Geometry check sheet. Reference: drawing and pictorial views, mm from the part's lowest x, y, z. A direction names the side the tool comes from. Coordinates: 2 decimals unless noted, no trailing zeros. Loops run counter-clockwise (first coordinate to the right, second up) from the corner with the lowest first, then second, coordinate; pieces in that order, holes last. Notation, with made-up numbers: (50.5, 57) -> (105.5, 57) arc R14 cw to (105.5, 84) -> close; hole circle Ø2 at (0, 59). An arc over 180 degrees is marked (long way). Answer as a JSON object with one key per item and string values.
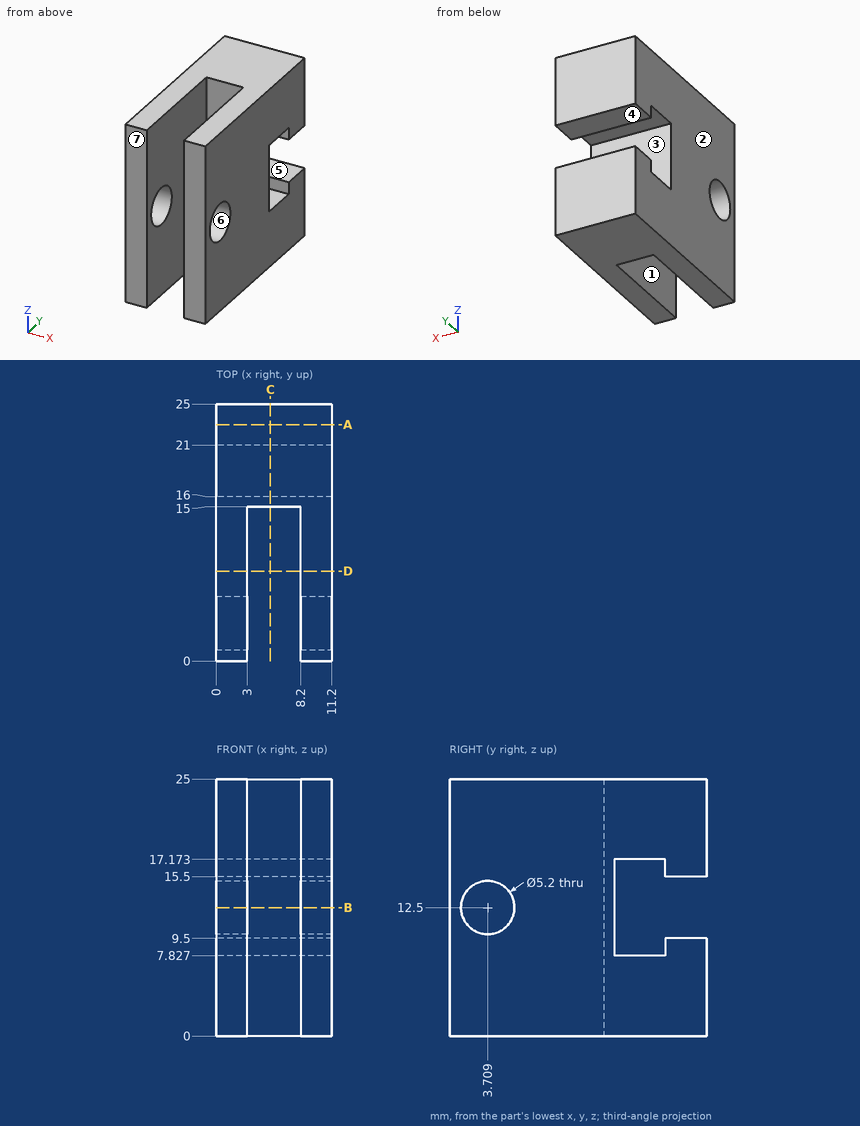
1. Section check B-B, the plane z = 12.5. Record the boundary of the cut face in (x, y), then the cut area to 3 significant figures.
Evaluation:
{"outline": "(0, 0) -> (3, 0) -> (3, 1.11) -> (0, 1.11) -> close; (0, 6.31) -> (3, 6.31) -> (3, 15) -> (8.2, 15) -> (8.2, 6.31) -> (11.2, 6.31) -> (11.2, 16) -> (0, 16) -> close; (8.2, 0) -> (11.2, 0) -> (11.2, 1.11) -> (8.2, 1.11) -> close", "area": "70.0 mm^2"}
2. Section check D-D, the plane y = 8.75. Record the boundary of the cut face in (x, z), then the cut area to 3 significant figures.
Evaluation:
{"outline": "(0, 0) -> (3, 0) -> (3, 25) -> (0, 25) -> close; (8.2, 0) -> (11.2, 0) -> (11.2, 25) -> (8.2, 25) -> close", "area": "150 mm^2"}
3. Section check A-A, the plane y = 23. Record the boundary of the cut face in (x, z).
Evaluation:
{"outline": "(0, 0) -> (11.2, 0) -> (11.2, 9.5) -> (0, 9.5) -> close; (0, 15.5) -> (11.2, 15.5) -> (11.2, 25) -> (0, 25) -> close"}
4. Section check C-C, the plane x = 5.25. Record the boundary of the cut face in (y, z), then the cut area to 3 significant figures.
Evaluation:
{"outline": "(15, 0) -> (25, 0) -> (25, 9.5) -> (21, 9.5) -> (21, 7.83) -> (16, 7.83) -> (16, 17.17) -> (21, 17.17) -> (21, 15.5) -> (25, 15.5) -> (25, 25) -> (15, 25) -> close", "area": "179 mm^2"}
5. Thickness scan on probe 1 along X at (y, z) = (9.75, 22.5); probe 2 along Z at (x, y) = (5.5, 16.5); probe 3 along Z at (x, y) = (9.5, 22.5). Record the ranges inside material, lowest first. Write a range as from..to.
Evaluation:
{"probe 1": "x = 0..3, 8.2..11.2", "probe 2": "z = 0..7.83, 17.17..25", "probe 3": "z = 0..9.5, 15.5..25"}
6. Mould release check, pull along Y, two halves, no side actions. Record for the marked faces 5, 6 and 7: released by +Y, released by -Y, zero draft, split by the parting line, or undercut.
Evaluation:
{"face 5": "zero draft", "face 6": "undercut", "face 7": "released by -Y"}
7. Depth check by flat-ended pin: P1, Ø5.5, axis at x = 4, y = 17.5, coming from the -Z side; P2, Ø0.8, axis at x = 4.5, z = 8.5, coming from the -Y side. Enter the tip coordinate at first touch or a pass-through.
Evaluation:
{"P1": "stops at z = 0", "P2": "stops at y = 15"}
8. Tool access check on the marked faces 1, 2, 3 and 4. Record the directions out of +Z, -Z, +X, -X, +Y, -Y that give a thin tool (end or side, any length) a straight path to the whole face; none if there is none.
Evaluation:
{"face 1": "+Z, -Z, -Y", "face 2": "+Z, -Z, -X, +Y, -Y", "face 3": "+X, -X", "face 4": "+X, -X, +Y"}
